Check sheet for the drawn part. Datum: minimum x, y, z corner. Units: mm. A direction names the side the tool comes from. Round coordinates to 2 decimals unless told otherwise and drop trailing zeros. Order: outer loops, then holes, each group sorted by start corner. A loop starts at its lowest first (then second) coordinate and runs counter-clockwise, first axis right, second up. Notation, with made-up numbers: (10.25, -1.75) - (23.25, -1.75) arc R4 cw to (23.25, 3.25) - close; hole circle Ø11 at (75.25, 34). An arc over 180 degrees is marked (long way). Write each question's results on one line, items separated by ' | '.
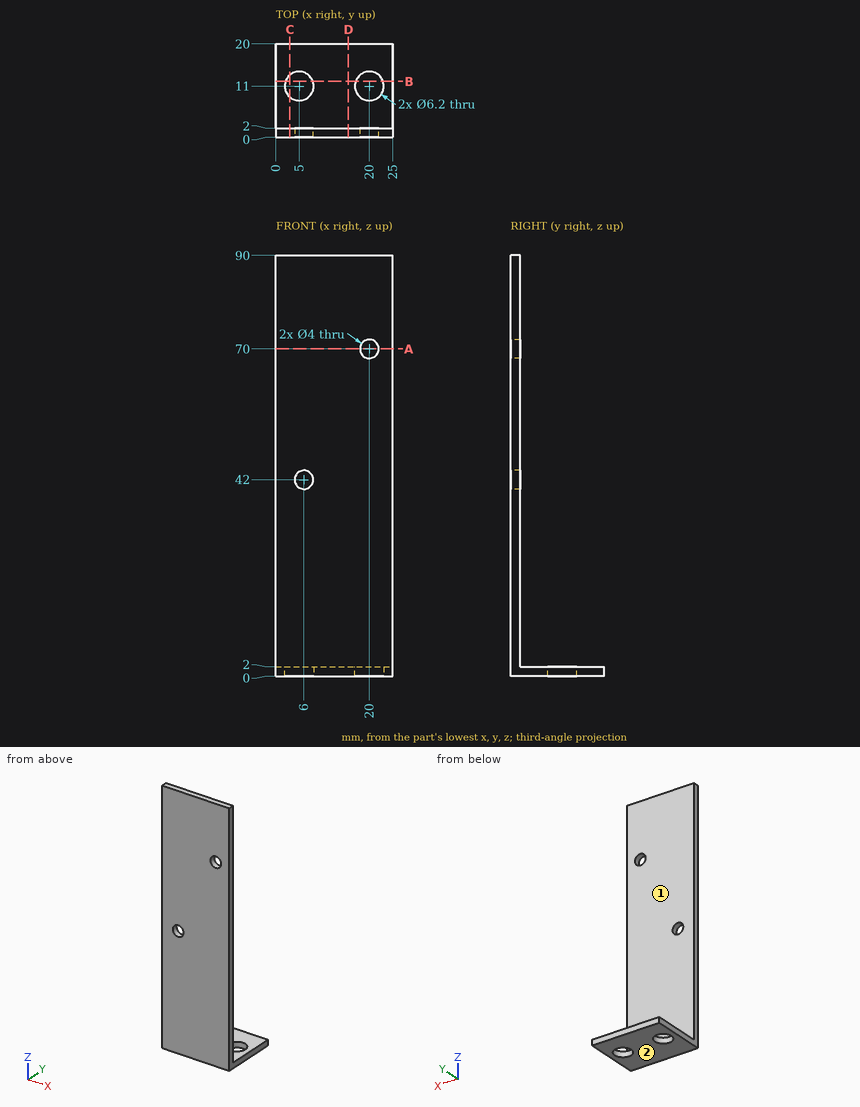
(1) Section check D-D (x = 15.5). Record the cut outline in (y, z).
Answers follow:
outline: (0, 0) - (20, 0) - (20, 2) - (2, 2) - (2, 90) - (0, 90) - close
(2) Access from +Z, -Z, +X, -X, +Y, -Y to the whole of each face (thin tool, end or side, straight path). Record for the marked faces 1 and 2.
Answers follow:
face 1: +Z, +X, -X, +Y | face 2: -Z, +X, -X, +Y, -Y
(3) Section check A-A (z = 70). Record the cut outline in (x, y), then the cut area to 3 significant figures.
Answers follow:
outline: (0, 0) - (18, 0) - (18, 2) - (0, 2) - close; (22, 0) - (25, 0) - (25, 2) - (22, 2) - close | area: 42.0 mm²
(4) Depth check by flat-ended pin: pin 1 Ø1 at (x, y) = (13, 12) entering from -Z; pin 2 Ø2.5 at (x, z) = (6, 42) entering from +Y; pin 3 Ø10 at (x, y) = (5, 11) entering from +Z. Enter the tip coordinate at first touch or a pass-through.
Answers follow:
pin 1: z = 0 | pin 2: through | pin 3: z = 2
(5) Section check B-B (y = 12). Record the cut outline in (x, z).
Answers follow:
outline: (0, 0) - (2.07, 0) - (2.07, 2) - (0, 2) - close; (7.93, 0) - (17.07, 0) - (17.07, 2) - (7.93, 2) - close; (22.93, 0) - (25, 0) - (25, 2) - (22.93, 2) - close
(6) Material ranges on line 1 (Y direction, x = 20, z = 0.75); line 2 (Z direction, x = 20, y = 0.55); line 3 (Z direction, x = 13.75, y = 9), recorded low to high.
Answers follow:
line 1: 0 to 7.9, 14.1 to 20 | line 2: 0 to 68, 72 to 90 | line 3: 0 to 2
(7) Section check C-C (x = 3). Record the cut outline in (y, z).
Answers follow:
outline: (0, 0) - (8.63, 0) - (8.63, 2) - (2, 2) - (2, 90) - (0, 90) - close; (13.37, 0) - (20, 0) - (20, 2) - (13.37, 2) - close
